from build123d import *

# Parameters (mm, degrees)
SKETCH_1_R      = 1.6
EXTRUDE_1_DEPTH = 5
FILLET_1_R      = 10
FILLET_2_R      = 3


with BuildPart() as part:
    # 草图1 → 凸台-拉伸1 (new body)
    with BuildSketch(Plane(origin=(0, 0, 0), x_dir=(1, 0, 0), z_dir=(0, 1, 0))):
        Polygon((0, -105), (-20, -105), (-20, 40), (181.865334795, 40), (181.865334795, 0), align=None)
        with Locations(Location((-10, -5, 0), (0, 0, 270))):
            Circle(SKETCH_1_R, mode=Mode.SUBTRACT)
        with Locations(Location((-10, -25, 0), (0, 0, 270))):
            Circle(SKETCH_1_R, mode=Mode.SUBTRACT)
        with Locations(Location((-10, -45, 0), (0, 0, 270))):
            Circle(SKETCH_1_R, mode=Mode.SUBTRACT)
        with Locations(Location((-10, 10, 0), (0, 0, 270))):
            Circle(SKETCH_1_R, mode=Mode.SUBTRACT)
        with Locations(Location((-10, 30, 0), (0, 0, 270))):
            Circle(SKETCH_1_R, mode=Mode.SUBTRACT)
        with Locations(Location((10, 30, 0), (0, 0, 270))):
            Circle(SKETCH_1_R, mode=Mode.SUBTRACT)
        with Locations(Location((10, 10, 0), (0, 0, 270))):
            Circle(SKETCH_1_R, mode=Mode.SUBTRACT)
        with Locations(Location((30, 10, 0), (0, 0, 270))):
            Circle(SKETCH_1_R, mode=Mode.SUBTRACT)
        with Locations(Location((-10, -65, 0), (0, 0, 270))):
            Circle(SKETCH_1_R, mode=Mode.SUBTRACT)
        with Locations(Location((-10, -85, 0), (0, 0, 270))):
            Circle(SKETCH_1_R, mode=Mode.SUBTRACT)
        with Locations(Location((50, 10, 0), (0, 0, 270))):
            Circle(SKETCH_1_R, mode=Mode.SUBTRACT)
        with Locations(Location((70, 10, 0), (0, 0, 270))):
            Circle(SKETCH_1_R, mode=Mode.SUBTRACT)
        with Locations(Location((90, 10, 0), (0, 0, 270))):
            Circle(SKETCH_1_R, mode=Mode.SUBTRACT)
        with Locations(Location((110, 10, 0), (0, 0, 270))):
            Circle(SKETCH_1_R, mode=Mode.SUBTRACT)
        with Locations(Location((130, 10, 0), (0, 0, 270))):
            Circle(SKETCH_1_R, mode=Mode.SUBTRACT)
        with Locations(Location((150, 10, 0), (0, 0, 270))):
            Circle(SKETCH_1_R, mode=Mode.SUBTRACT)
        with Locations(Location((170, 10, 0), (0, 0, 270))):
            Circle(SKETCH_1_R, mode=Mode.SUBTRACT)
        with Locations(Location((50, 30, 0), (0, 0, 270))):
            Circle(SKETCH_1_R, mode=Mode.SUBTRACT)
        with Locations(Location((70, 30, 0), (0, 0, 270))):
            Circle(SKETCH_1_R, mode=Mode.SUBTRACT)
        with Locations(Location((90, 30, 0), (0, 0, 270))):
            Circle(SKETCH_1_R, mode=Mode.SUBTRACT)
        with Locations(Location((110, 30, 0), (0, 0, 270))):
            Circle(SKETCH_1_R, mode=Mode.SUBTRACT)
        with Locations(Location((130, 30, 0), (0, 0, 270))):
            Circle(SKETCH_1_R, mode=Mode.SUBTRACT)
        with Locations(Location((150, 30, 0), (0, 0, 270))):
            Circle(SKETCH_1_R, mode=Mode.SUBTRACT)
        with Locations(Location((170, 30, 0), (0, 0, 270))):
            Circle(SKETCH_1_R, mode=Mode.SUBTRACT)
        with Locations(Location((30, 30, 0), (0, 0, 270))):
            Circle(SKETCH_1_R, mode=Mode.SUBTRACT)
        Polygon((0, -76.132486541), (0, 0), (131.865334795, 0), align=None, mode=Mode.SUBTRACT)
    extrude(amount=EXTRUDE_1_DEPTH)

    # 圆角1
    fillet_1_edges = [part.edges().sort_by_distance(p)[0] for p in [
        (0, 2.5, 0),
        (0, 2.5, 76.132486541),
        (131.865334795, 2.5, 0),
    ]]
    fillet(fillet_1_edges, radius=FILLET_1_R)

    # 圆角2
    fillet_2_edges = [part.edges().sort_by_distance(p)[0] for p in [
        (-20, 2.5, 105),
        (-20, 2.5, -40),
        (181.865334795, 2.5, -40),
        (181.865334795, 2.5, 0),
        (0, 2.5, 105),
    ]]
    fillet(fillet_2_edges, radius=FILLET_2_R)


solid = part.part
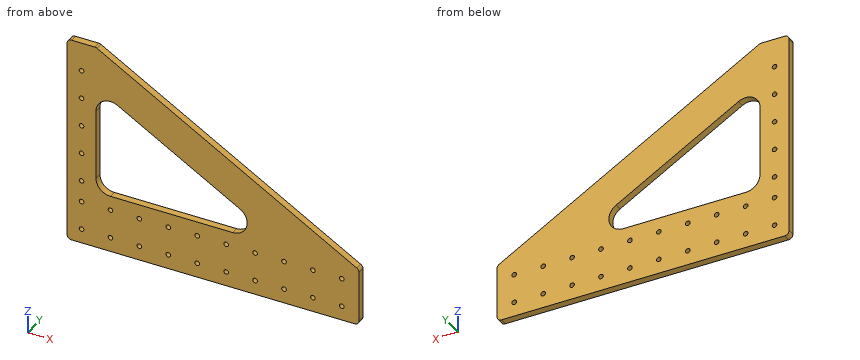
Build history of the part. All positions in model axes, mm. Give positions to 0.01 mm unless a question says otherwise; leave off trailing zeros. Loops run counter-clockwise (first coordinate to the right, second up) from the corner with the lowest first, then second, coordinate; pieces in that order, holes last. Notation, with made-up numbers: (-9.75, 57.25) - (17.25, 57.25) arc R25 cw to (17.25, 90.25) - close; hole circle Ø5 at (85, 72). An arc over 180 degrees is marked (long way). Write item = value, one per line. Start each with the question number.
1) Band-saw the part on A-A on z = 33.5. Give the cut face in (x, y), plus the area to 3 significant figures.
2) Drop flat-ended pins along their axis: pin 1 Ø2.5 at (x, z) = (110, -30) entering from +Y; pin 2 Ø1 at (y, z) = (4.5, 78) entering from +X. Give the stop position or say it passes through.
3) Band-saw the part on D-D on x = 160. Give the cut face in (y, z), plus the area to 3 significant figures.
4) Probe probe 1 along Z at (x, y) = (70, 4.05); probe 2 along X at (y, z) = (3.15, 65); probe 3 along Z at (x, y) = (170, 2.6). List the from-to ranges inside material, lowest first. Write a range as from..to.
5) Band-saw the part on B-B on y = 2.05. Count the separate pieces of the cut face and the enclosed holes in it, plus the area to 3 significant figures.
6) Band-saw the part on C-C on x = 117.5. Give the cut face in (y, z).
Final values:
q1.outline = (-20, 0) - (0, 0) - (0, 5) - (-20, 5) - close; (73.84, 0) - (123.84, 0) - (123.84, 5) - (73.84, 5) - close
q1.area = 350 mm²
q2.pin_1 = through
q2.pin_2 = 47.63
q3.outline = (0, -40) - (5, -40) - (5, 12.62) - (0, 12.62) - close
q3.area = 263 mm²
q4.probe_1 = -40..-31.6, -28.4..-11.6, -8.4..0, 35.72..64.59
q4.probe_2 = -20..-11.6, -8.4..2.14, 19.28..69.28
q4.probe_3 = -40..-31.6, -28.4..-11.6, -8.4..6.85
q5.separate_pieces = 1
q5.enclosed_holes = 26
q5.area = 14,800 mm²
q6.outline = (0, -40) - (5, -40) - (5, 37.16) - (0, 37.16) - close
